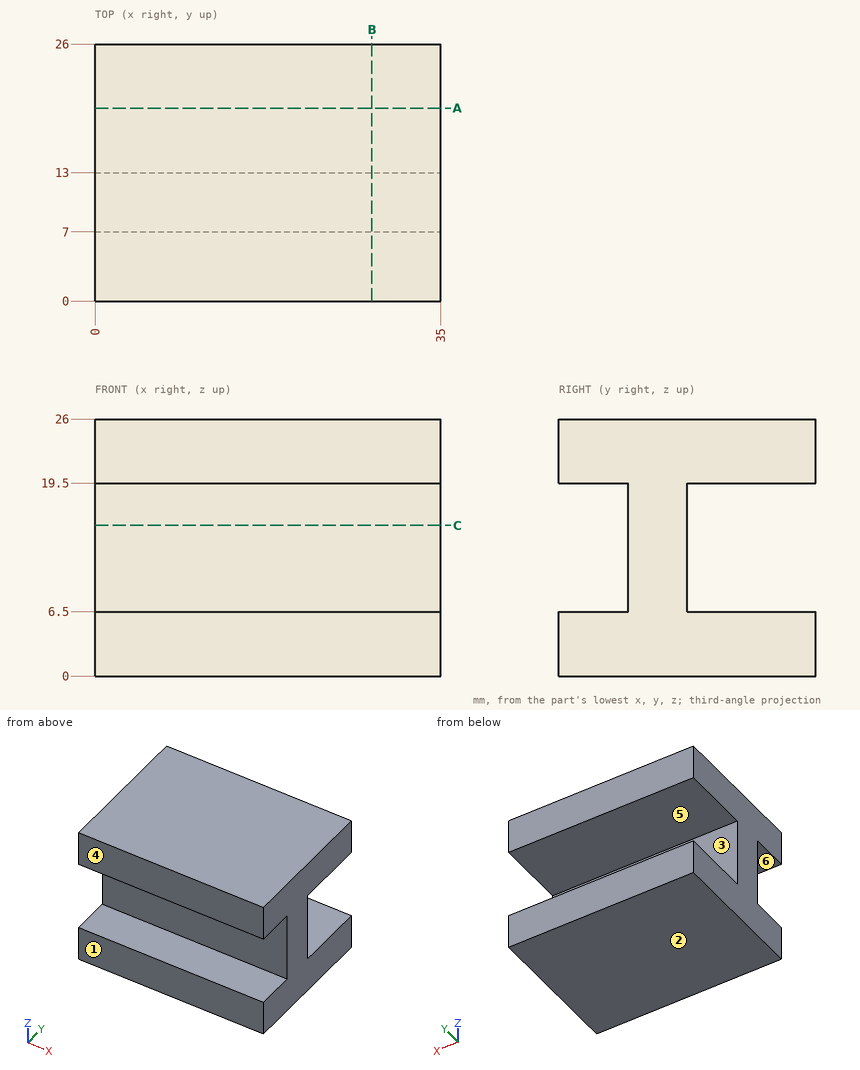
Geometry: see drawing. Coordinates: mm, zero at the bounding-box minimum. A direction names the side the tool comes from. Round coordinates to 2 decimals unless told otherwise and drop trailing zeros. Loops run counter-clockwise (first coordinate to the right, second up) from the corner with the lowest first, then second, coordinate; pieces in that order, holes last. Notation, with made-up numbers: (88, 39.25) -> (105, 39.25) arc R27 ccw to (105, 78.25) -> close; hole circle Ø5 at (72.25, -23.5). An arc over 180 degrees is marked (long way). One line per question, with ' | ' between items. Start each with the question number.
1. Mould query, pull axis Z, two halves, no side actions, for the marked faces 1, 2 and 3. Classes: pulls with the +Z half, pulls with the -Z half, needs draft (parallel to the pull), parting line crosses it, or undercut.
2. Section B-B on x = 28. Output: boundary loops of the cut face in (y, z), and give its area (3 significant figures).
3. Section C-C on z = 15.25. Output: boundary loops of the cut face in (x, y), and give its area (3 significant figures).
4. Contact query for flat-ended pins moving along their axis: pin 1 (4 mm diameter, centred on x = 21, z = 11, fed in from -Y); pin 2 (6 mm diameter, centred on x = 9.5, z = 11.5, fed in from +Y). Output: stop coordinate, or through.
5. Line query: line 1 along Z through (x, y) = (24.5, 16.75); line 2 along Y through (x, z) = (24.5, 10.25). Output: solid intervals per line, ascending. Write a range as [from, to].
6. Set-up query: the marked faces 4, 5 and 6. Return all of +Z, -Z, +X, -X, +Y, -Y with unobstructed straight access to the full face (end or side cutting, diameter ignored); none if empty.
7. Section A-A on y = 19.5. Output: boundary loops of the cut face in (x, z).
Returned:
1) face 1: needs draft | face 2: pulls with the -Z half | face 3: undercut
2) outline: (0, 0) -> (26, 0) -> (26, 6.5) -> (13, 6.5) -> (13, 19.5) -> (26, 19.5) -> (26, 26) -> (0, 26) -> (0, 19.5) -> (7, 19.5) -> (7, 6.5) -> (0, 6.5) -> close | area: 416 mm2
3) outline: (0, 7) -> (35, 7) -> (35, 13) -> (0, 13) -> close | area: 210 mm2
4) pin 1: stops at y = 7 | pin 2: stops at y = 13
5) line 1: z = [0, 6.5], [19.5, 26] | line 2: y = [7, 13]
6) face 4: +Z, -Z, +X, -X, -Y | face 5: +X, -X, +Y | face 6: +X, -X, -Y
7) outline: (0, 0) -> (35, 0) -> (35, 6.5) -> (0, 6.5) -> close; (0, 19.5) -> (35, 19.5) -> (35, 26) -> (0, 26) -> close
